The model under review builds one solid part; all positions refer to its coordinate system, in mm. Face numbers are marked on the shaded views. A direction names the side the tool comes from. Round coordinates to 2 decimals unless told otherwise and drop trailing zeros. Order: outer loops, then holes, each group sorted by start corner. A loop starts at its lowest first (then second) coordinate and runs counter-clockwise, first axis right, second up. Notation, with made-up numbers: (-4, 64) - (13, 64) arc R8 ccw to (13, 72) - close; hole circle Ø3 at (43, 39). An arc over 180 degrees is marked (long way). One line per question, with ' | ' between items. Start each with the question number.
Item 1: Insertion check: pin 1 Ø1.5 at (x, z) = (19.5, -5) entering from +Y; pin 2 Ø5 at (x, z) = (-20, 11.825) entering from +Y; pin 3 Ø1.5 at (x, y) = (-21, 55) entering from -Z. Each pin has a flat end and moves straight along its axis. Give the tip position at first contact, or say it passes through.
Item 2: Add section A-A on y = 63. State the section outline as (x, z) points.
Item 3: Tool access review of the marked faces 1 and 2: name each direction out of +Z, -Z, +X, -X, +Y, -Y from which nothing blocks a thin tool from reaching the whole face with its end or side.
Item 4: Add section C-C on y = 23. State the section outline as (x, z) points, and give its area (3 significant figures).
Item 5: For L1, parallel to Y at x = 20, z = -11.7; L2, parallel to Y at x = -20, z = -18.65; L3, parallel to Z at x = 20, y = 67.4, list the stretches that pass through material, from the lowest coordinate up. Write a range as [from, to].
Item 6: Add section B-B on x = -12.5. State the section outline as (y, z) points, and give its area (3 significant figures).
from build123d import *

# Parameters (mm, degrees)
SKETCH1_W                               = 60
SKETCH1_H                               = 40
BOSS_EXTRUDE1_DEPTH                     = 70
SKETCH2_W                               = 15
SKETCH2_H                               = 61.5
CUT_EXTRUDE1_DEPTH                      = 90
CSK_FOR_M4_SFHCS1_D                     = 4.5
CSK_FOR_M4_SFHCS1_CSINK_D               = 8.96
CSK_FOR_M4_SFHCS1_CSINK_ANGLE           = 90
CBORE_FOR_M5_HEX_HEAD_BOLT1_D           = 4.5
CBORE_FOR_M5_HEX_HEAD_BOLT1_DEPTH       = 10
CBORE_FOR_M5_HEX_HEAD_BOLT1_CBORE_D     = 5
CBORE_FOR_M5_HEX_HEAD_BOLT1_CBORE_DEPTH = 4.2
CBORE_FOR_M5_HEX_HEAD_BOLT1_TIP         = 1.351936393
CBORE_FOR_M5_HEX_HEAD_BOLT2_D           = 4.5
CBORE_FOR_M5_HEX_HEAD_BOLT2_DEPTH       = 10
CBORE_FOR_M5_HEX_HEAD_BOLT2_CBORE_D     = 5
CBORE_FOR_M5_HEX_HEAD_BOLT2_CBORE_DEPTH = 4.2
CBORE_FOR_M5_HEX_HEAD_BOLT2_TIP         = 1.351936393
CHAMFER2_SIZE                           = 2


with BuildPart() as part:
    # Sketch1 → Boss-Extrude1 (new body)
    with BuildSketch(Plane(origin=(0, 0, 0), x_dir=(1, 0, 0), z_dir=(0, 1, 0))):
        Rectangle(SKETCH1_W, SKETCH1_H)
    extrude(amount=BOSS_EXTRUDE1_DEPTH)

    # Sketch2 → Cut-Extrude1 (cut)
    with BuildSketch(Plane(origin=(30, 0, 0), x_dir=(0, 0, -1), z_dir=(1, 0, 0))):
        with Locations((-12.5, 39.25)):
            Rectangle(SKETCH2_W, SKETCH2_H)
    extrude(amount=-CUT_EXTRUDE1_DEPTH, mode=Mode.SUBTRACT)

    # CSK for M4 SFHCS1 (through all)
    with Locations(Plane(origin=(0, 8.5, 0), x_dir=(1, 0, 0), z_dir=(0, 1, 0))):
        with Locations((-20, -11.825), (20, -11.825)):
            CounterSinkHole(CSK_FOR_M4_SFHCS1_D / 2, CSK_FOR_M4_SFHCS1_CSINK_D / 2, counter_sink_angle=CSK_FOR_M4_SFHCS1_CSINK_ANGLE)

    # CBORE for M5 Hex Head Bolt1
    with Locations(Plane(origin=(0, 0, -20), x_dir=(-1, 0, 0), z_dir=(0, 0, -1))):
        with Locations((20, 55), (-20, 15), (-20, 55), (20, 15)):
            CounterBoreHole(CBORE_FOR_M5_HEX_HEAD_BOLT1_D / 2, CBORE_FOR_M5_HEX_HEAD_BOLT1_CBORE_D / 2, CBORE_FOR_M5_HEX_HEAD_BOLT1_CBORE_DEPTH, depth=CBORE_FOR_M5_HEX_HEAD_BOLT1_DEPTH)
            with Locations((0, 0, -(CBORE_FOR_M5_HEX_HEAD_BOLT1_DEPTH + CBORE_FOR_M5_HEX_HEAD_BOLT1_TIP / 2))):  # 118° drill point
                Cone(0, CBORE_FOR_M5_HEX_HEAD_BOLT1_D / 2, CBORE_FOR_M5_HEX_HEAD_BOLT1_TIP, mode=Mode.SUBTRACT)

    # CBORE for M5 Hex Head Bolt2
    with Locations(Plane(origin=(0, 70, 0), x_dir=(1, 0, 0), z_dir=(0, 1, 0))):
        with Locations((-20, 5), (20, 5)):
            CounterBoreHole(CBORE_FOR_M5_HEX_HEAD_BOLT2_D / 2, CBORE_FOR_M5_HEX_HEAD_BOLT2_CBORE_D / 2, CBORE_FOR_M5_HEX_HEAD_BOLT2_CBORE_DEPTH, depth=CBORE_FOR_M5_HEX_HEAD_BOLT2_DEPTH)
            with Locations((0, 0, -(CBORE_FOR_M5_HEX_HEAD_BOLT2_DEPTH + CBORE_FOR_M5_HEX_HEAD_BOLT2_TIP / 2))):  # 118° drill point
                Cone(0, CBORE_FOR_M5_HEX_HEAD_BOLT2_D / 2, CBORE_FOR_M5_HEX_HEAD_BOLT2_TIP, mode=Mode.SUBTRACT)

    # Chamfer2
    chamfer2_edges = [part.edges().sort_by_distance(p)[0] for p in [
        (0, 70, 5),
        (0, 8.5, 20),
        (0, 0, 20),
        (0, 0, -20),
        (0, 70, -20),
    ]]
    chamfer(chamfer2_edges, length=CHAMFER2_SIZE)


solid = part.part
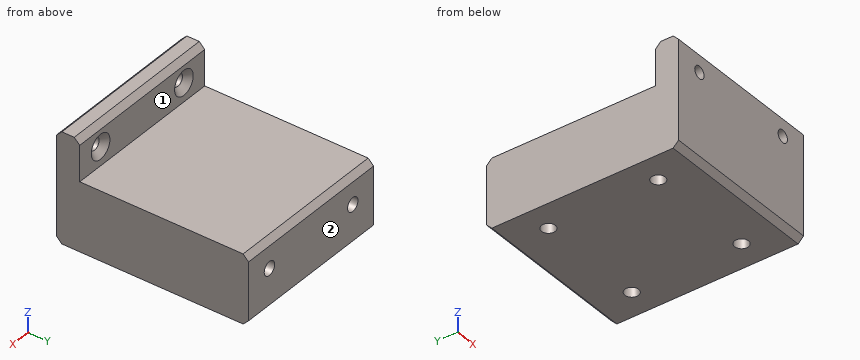
Determined:
1) pin 1: y = 59.4 | pin 2: y = 6.52 | pin 3: z = -9.7
2) outline: (-30, -20) - (30, -20) - (30, 5) - (-30, 5) - close; hole circle Ø4.5 at (-20, -5); hole circle Ø4.5 at (20, -5)
3) face 1: +Z, +X, -X, +Y | face 2: +Z, -Z, +X, -X, +Y
4) outline: (-30, -20) - (30, -20) - (30, 5) - (-30, 5) - close | area: 1,500 mm2
5) L1: [0, 12.75], [17.25, 52.75], [57.25, 70] | L2: [0.65, 12.5], [17.5, 52.5], [57.5, 69.35] | L3: [-20, -7.5], [-2.5, 5]
6) outline: (0, -18) - (2, -20) - (68, -20) - (70, -18) - (70, 3) - (68, 5) - (8.5, 5) - (8.5, 18) - (6.5, 20) - (2, 20) - (0, 18) - close | area: 1,870 mm2
